Read the model definition and answer for the solid it produces. Units are mm, in the model's axes. A direction names the side the tool comes from. Give positions to 0.01 mm unless a question says otherwise; leave off trailing zeros. Order: outer loops, then holes, each group sorted by start corner. A loop starts at its lowest first (then second) coordinate and runs counter-clockwise, first axis right, second up.
Item 1: Which of the six approach directions +Z, -Z, +X, -X, +Y, -Y give full straight-line access (tool end or side, diameter ignored) to faces 5 (the face through (101.549, -0.444, 16.084)), 6 (the face through (31, -0.9, -69))?
Item 2: Find the intervals of material crossed by line 1 along X through (y, z) = (-0.5, -61.5); line 2 along X through (y, z) = (-0.05, -85); line 3 along X through (y, z) = (-0.15, -54.5), in increasing order.
Item 3: A cutting plane is placed at A-A (x = 0). Write down the section's boundary in (y, z).
Item 4: The mould has two halves that part along X. Classify faces 1 (the face through (31, 0, -69)), 2 (the face through (17.809, -0.444, -72.855)), 3 (the face through (-99.88, -0.44, -21.23)), 4 (the face through (18.96, -0.44, -77.72)): +X half, -X half, draft (parallel to the pull), parting line (faces both ways), or undercut.
Item 5: Given pin 1 Ø8 at (x, z) = (63, -61) entering from -Y, flat-ended and moving along its own axis, determine where the tip first touches the part or whether it passes through.
Item 6: A cutting plane is placed at C-C (y = -0.2). Write down the section's boundary in (x, z), plus the area to 3 significant figures.
Item 7: A cutting plane is placed at D-D (z = -56.5). Write down the section's boundary in (x, y), plus the area to 3 significant figures.
Item 8: A cutting plane is placed at B-B (z = 0). Write down the section's boundary in (x, y), plus the area to 3 significant figures.
from build123d import *

# Parameters (mm, degrees)
BASE_FLANGE1_DEPTH = 0.9


# Sheet-metal steps are written as plain solids
with BuildPart() as part:
    # Sketch1 → Base-Flange1 (new body)
    with BuildSketch(Plane(origin=(0, 0, 0), x_dir=(1, 0, 0), z_dir=(0, 1, 0))):
        with BuildLine():
            Line((-76.23906038, 16.205112539), (-124.190081684, 26.397416756))
            ThreePointArc((-124.190081684, 26.397416756), (-126.101482372, 27.727775186), (-126.485236689, 30.024738131))
            ThreePointArc((-126.485236689, 30.024738131), (28.137149812, 126.918480926), (127.323557594, -26.243316894))
            ThreePointArc((127.323557594, -26.243316894), (126.005019582, -28.162890715), (123.710468487, -28.560812083))
            Line((123.710468487, -28.560812083), (75.944630591, -17.53319949))
            ThreePointArc((75.944630591, -17.53319949), (74.106388046, -16.248487893), (73.672580533, -14.048162785))
            ThreePointArc((73.672580533, -14.048162785), (16.232971045, 73.222200534), (-72.707043565, 18.403418598))
            ThreePointArc((-72.707043565, 18.403418598), (-74.030104265, 16.592581795), (-76.23906038, 16.205112539))
        make_face()
        with BuildLine():
            Line((-76.900935675, 22.050988465), (-120.157711992, 34.454669477))
            ThreePointArc((-120.157711992, 34.454669477), (27.054951742, 122.03700089), (123.461042574, -19.55430813))
            Line((123.461042574, -19.55430813), (79.015067248, -12.514757203))
            ThreePointArc((79.015067248, -12.514757203), (17.315169115, 78.10368057), (-76.900935675, 22.050988465))
        make_face(mode=Mode.SUBTRACT)
    extrude(amount=-BASE_FLANGE1_DEPTH)


solid = part.part
Response values:
1. face 5: +Y, -Y
1. face 6: +Z, -Z, +X, -X, -Y
2. line 1: x = -114.53 to -108.82, -51.16 to -42.93, 42.93 to 51.16, 108.82 to 114.53
2. line 2: x = -98.36 to -91.65, 91.65 to 98.36
2. line 3: x = -118.02 to -112.49, -58.56 to -51.52, 51.52 to 58.56, 112.49 to 118.02
3. outline: (-0.9, -130) - (0, -130) - (0, -125) - (-0.9, -125) - close; (-0.9, -80) - (0, -80) - (0, -75) - (-0.9, -75) - close
4. face 1: draft
4. face 2: undercut
4. face 3: -X half
4. face 4: undercut
5. pin 1: passes through
6. outline: (-126.49, -30.02) arc R130 ccw to (127.32, 26.24) arc R3 ccw to (123.71, 28.56) - (75.94, 17.53) arc R3 ccw to (73.67, 14.05) arc R75 cw to (-72.71, -18.4) arc R3 ccw to (-76.24, -16.21) - (-124.19, -26.4) arc R3 ccw to start; hole (-120.16, -34.45) arc R125 ccw to (123.46, 19.55) - (79.02, 12.51) arc R80 cw to (-76.9, -22.05) - close
6. area: 3,870 mm2
7. outline: (-117.08, -0.9) - (-111.5, -0.9) - (-111.5, 0) - (-117.08, 0) - close; (-56.64, -0.9) - (-49.32, -0.9) - (-49.32, 0) - (-56.64, 0) - close; (49.32, -0.9) - (56.64, -0.9) - (56.64, 0) - (49.32, 0) - close; (111.5, -0.9) - (117.08, -0.9) - (117.08, 0) - (111.5, 0) - close
7. area: 23.2 mm2
8. outline: (75, -0.9) - (80, -0.9) - (80, 0) - (75, 0) - close; (125, -0.9) - (130, -0.9) - (130, 0) - (125, 0) - close
8. area: 9.00 mm2
